Part model, mm, in its own coordinate system. Face numbers are marked on the shaded views. A direction names the side the tool comes from. Coordinates: 2 decimals unless noted, no trailing zeros. Loops run counter-clockwise (first coordinate to the right, second up) from the corner with the lowest first, then second, coordinate; pieces in that order, holes last. Notation, with made-up numbers: (72, 83) - (117, 83) arc R21 ccw to (117, 97) - close; hole circle Ø6 at (-19, 39.25). An arc over 180 degrees is marked (long way). Use a Markdown table: item, result. Add a question column.
1) Pull direction X, two halves, no side cores. Call the marked faces 3, 4 and 5: +X half, -X half, draft (parallel to the pull), parting line (faces both ways), or undercut.
2) Band-saw the part on C-C (z = 1.25). Give the cut face in (x, y).
3) Tool access for the marked faces 1 and 2: list every direction of +Z, -Z, +X, -X, +Y, -Y with a clear straight run to the whole face (end or side of a thin tool).
4) Band-saw the part on A-A (y = 0). Give the cut face in (x, z), plus the area to 3 significant figures.
5) Band-saw the part on D-D (y = 1.5). Give the cut face in (x, z), plus the area to 3 significant figures.
6) Probe probe 1 along Y at (x, z) = (0, 10.5); probe 2 along Y at (x, z) = (0, 1.9); probe 3 along Z at (x, y) = (-1.5, -0.5). List the from-to ranges inside material, lowest first. Write a range as [from, to].
7) Drop flat-ended pins along their axis: P1, Ø1.5, axis at y = 1, z = 4.5, coming from the -X side; P2, Ø4, axis at x = 0, y = 0, coming from the +Z side; P3, Ø2.5, axis at x = 0.5, y = -0.5, coming from the -Z side; P4, Ø1.8, axis at x = 0, y = 0, coming from the -Z side. Give the stop position or say it passes through.
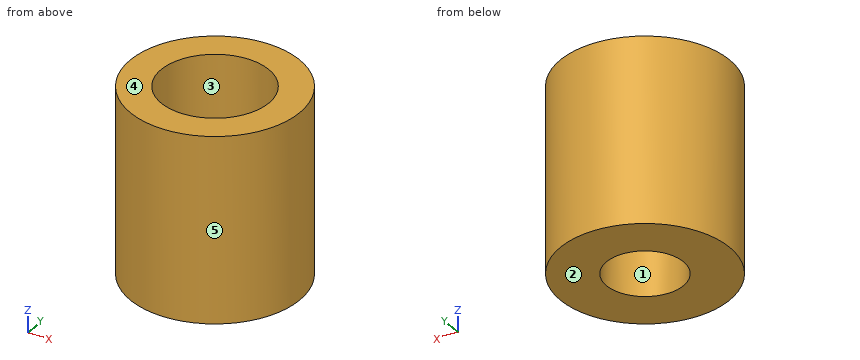
from build123d import *

# Parameters (mm, degrees)
SKETCH1_R           = 5.5
SKETCH1_R_2         = 2.5
BOSS_EXTRUDE1_DEPTH = 20
BOSS_EXTRUDE2_START = -17
SKETCH2_R           = 2.5
BOSS_EXTRUDE2_DEPTH = 2
SKETCH3_R           = 1
CUT_EXTRUDE1_DEPTH  = 2
SKETCH4_R           = 3.5
CUT_EXTRUDE3_DEPTH  = 15
SKETCH5_R           = 6.684025948
CUT_EXTRUDE4_DEPTH  = 8


with BuildPart() as part:
    # Sketch1 → Boss-Extrude1 (new body)
    with BuildSketch(Plane.XY):
        Circle(SKETCH1_R)
        Circle(SKETCH1_R_2, mode=Mode.SUBTRACT)
    extrude(amount=BOSS_EXTRUDE1_DEPTH)

    # Sketch2 → Boss-Extrude2 (add)
    with BuildSketch(Plane.XY.offset(20).offset(BOSS_EXTRUDE2_START)):
        Circle(SKETCH2_R)
    extrude(amount=BOSS_EXTRUDE2_DEPTH)

    # Sketch3 → Cut-Extrude1 (cut)
    with BuildSketch(Plane.XY.offset(5)):
        Circle(SKETCH3_R)
    extrude(amount=-CUT_EXTRUDE1_DEPTH, mode=Mode.SUBTRACT)

    # Sketch4 → Cut-Extrude3 (cut)
    with BuildSketch(Plane.XY.offset(20)):
        Circle(SKETCH4_R)
    extrude(amount=-CUT_EXTRUDE3_DEPTH, mode=Mode.SUBTRACT)

    # Sketch5 → Cut-Extrude4 (cut)
    with BuildSketch(Plane.XY.offset(20)):
        Circle(SKETCH5_R)
    extrude(amount=-CUT_EXTRUDE4_DEPTH, mode=Mode.SUBTRACT)


solid = part.part
Answer block:
| question | item | result |
|---|---|---|
| 1 | face 3 | undercut |
| 1 | face 4 | draft |
| 1 | face 5 | parting line |
| 2 | outline | circle Ø11 at (0, 0); hole circle Ø5 at (0, 0) |
| 3 | face 1 | -Z |
| 3 | face 2 | -Z, +X, -X, +Y, -Y |
| 4 | outline | (-5.5, 0) - (-2.5, 0) - (-2.5, 3) - (-1, 3) - (-1, 5) - (-3.5, 5) - (-3.5, 12) - (-5.5, 12) - close; (1, 3) - (2.5, 3) - (2.5, 0) - (5.5, 0) - (5.5, 12) - (3.5, 12) - (3.5, 5) - (1, 5) - close |
| 4 | area | 64.0 mm2 |
| 5 | outline | (-5.29, 0) - (-2, 0) - (-2, 3) - (2, 3) - (2, 0) - (5.29, 0) - (5.29, 12) - (3.16, 12) - (3.16, 5) - (-3.16, 5) - (-3.16, 12) - (-5.29, 12) - close |
| 5 | area | 70.7 mm2 |
| 6 | probe 1 | [-5.5, -3.5], [3.5, 5.5] |
| 6 | probe 2 | [-5.5, -2.5], [2.5, 5.5] |
| 6 | probe 3 | [3, 5] |
| 7 | P1 | x = -5.49 |
| 7 | P2 | z = 5 |
| 7 | P3 | z = 3 |
| 7 | P4 | through |
